Model file for the job. Use its own axes, mm. Face numbers are marked on the shaded views. A direction names the side the tool comes from. Round coordinates to 2 decimals unless told otherwise and drop trailing zeros. Loops run counter-clockwise (first coordinate to the right, second up) from the corner with the lowest first, then second, coordinate; pieces in that order, holes last. Notation, with made-up numbers: (60.25, -21) - (100.25, -21) arc R20 ccw to (100.25, 0) - close; hole circle Ø1 at (-16, 32.5). An arc over 180 degrees is marked (long way). Use one line per item in the form item = value.
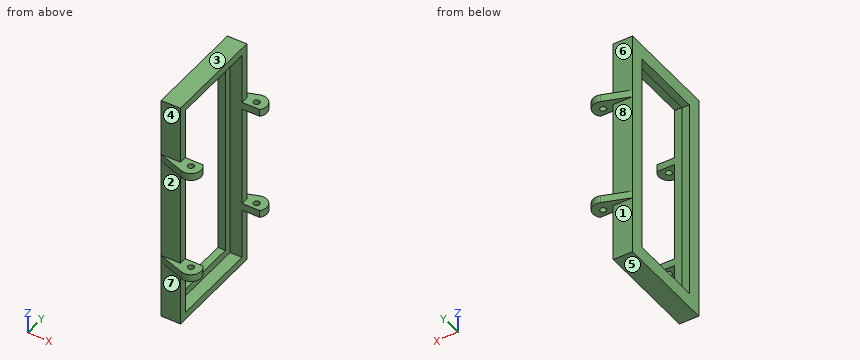
from build123d import *

# Parameters (mm, degrees)
SKETCH_1_W               = 114.4
SKETCH_1_H               = 50.4
SKETCH_1_W_2             = 107.2
SKETCH_1_H_2             = 43.2
SKETCH_1_W_3             = 100
SKETCH_1_H_3             = 36
EXTRUDE_1_DEPTH          = 3.6
SKETCH_1_3_W             = 114.4
SKETCH_1_3_H             = 50.4
SKETCH_1_3_W_2           = 107.2
SKETCH_1_3_H_2           = 43.2
EXTRUDE_2_DEPTH          = 9.5
EXTRUDE_START            = 25
SKETCH_2_R               = 1.5
EXTRUDE_3_DEPTH          = 3.6
MIRROR_START             = 25
MIRROR_2_COPY_1_SKETCH_R = 1.5
MIRROR_2_COPY_1_DEPTH    = 3.6


with BuildPart() as part:
    # Sketch 1 → Extrude 1 (new body)
    # profile 1 of 2: a face of its own
    with BuildSketch(Plane(origin=(0, 0, 0), x_dir=(0, 0, -1), z_dir=(1, 0, 0))):
        Rectangle(SKETCH_1_W, SKETCH_1_H)
        Rectangle(SKETCH_1_W_2, SKETCH_1_H_2, mode=Mode.SUBTRACT)
    # profile 2 of 2: a face of its own
    with BuildSketch(Plane(origin=(0, 0, 0), x_dir=(0, 0, -1), z_dir=(1, 0, 0))):
        Rectangle(SKETCH_1_W_2, SKETCH_1_H_2)
        Rectangle(SKETCH_1_W_3, SKETCH_1_H_3, mode=Mode.SUBTRACT)
    extrude(amount=EXTRUDE_1_DEPTH)

    # Sketch 1_3 → Extrude 2 (add)
    with BuildSketch(Plane(origin=(0, 0, 0), x_dir=(0, 0, -1), z_dir=(1, 0, 0))):
        Rectangle(SKETCH_1_3_W, SKETCH_1_3_H)
        Rectangle(SKETCH_1_3_W_2, SKETCH_1_3_H_2, mode=Mode.SUBTRACT)
    extrude(amount=EXTRUDE_2_DEPTH)

    # Sketch 2 → Extrude 3 (add)
    with BuildSketch(Plane.XY.offset(EXTRUDE_START)):
        with BuildLine():
            Line((12.840920286, 29.716720736), (0, 25.2))
            Line((0, 25.2), (0, 21.6))
            Line((0, 21.6), (9.5, 21.6))
            Line((9.5, 21.6), (18.166060556, 21.6))
            ThreePointArc((18.166060556, 21.6), (18.680583919, 27.74275739), (12.840920286, 29.716720736))
        make_face()
        with Locations((14.5, 25)):
            Circle(SKETCH_2_R, mode=Mode.SUBTRACT)
    extrude_3 = extrude(amount=EXTRUDE_3_DEPTH)

    # Mirror 1: Extrude 3 across plane
    add(extrude_3.mirror(Plane.XY))

    # Mirror 2: Extrude 3 across plane
    add(extrude_3.mirror(Plane.ZX))

    # Mirror 2 copy 1 sketch → Mirror 2 copy 1 (add)
    with BuildSketch(Plane(origin=(0, 0, 0), x_dir=(1, 0, 0), z_dir=(0, 0, -1)).offset(MIRROR_START)):
        with BuildLine():
            Line((12.840920286, 29.716720736), (0, 25.2))
            Line((0, 25.2), (0, 21.6))
            Line((0, 21.6), (9.5, 21.6))
            Line((9.5, 21.6), (18.166060556, 21.6))
            ThreePointArc((18.166060556, 21.6), (18.680583919, 27.74275739), (12.840920286, 29.716720736))
        make_face()
        with Locations((14.5, 25)):
            Circle(MIRROR_2_COPY_1_SKETCH_R, mode=Mode.SUBTRACT)
    extrude(amount=MIRROR_2_COPY_1_DEPTH)


solid = part.part
1. Cut at B-B, the plane x = 14.5. Give the number of separate pieces and of enclosed holes in the cut face, plus the area to 3 significant figures.
Geometry check:
separate_pieces = 8
enclosed_holes = 0
area = 77.8 mm^2
2. Pull direction Z, two halves, no side cores. Call the marked faces 1, 2 and 3: +Z half, -Z half, draft (parallel to the pull), parting line (faces both ways), or undercut.
Geometry check:
face_1 = draft
face_2 = undercut
face_3 = +Z half
3. Wall check: probe 1 along Y at (x, z) = (14.5, -25.95); probe 2 along Z at (x, y) = (1.25, 10); probe 3 along Y at (x, z) = (4, -13). Give the ranges that are in metal, low to high.
Geometry check:
probe_1 = -30 to -26.5, -23.5 to -21.6, 21.6 to 23.5, 26.5 to 30
probe_2 = -57.2 to -50, 50 to 57.2
probe_3 = -25.2 to -21.6, 21.6 to 25.2
4. Tool access for the marked faces 4, 5, 6, 7 and 8: list every direction of +Z, -Z, +X, -X, +Y, -Y with a clear straight run to the whole face (end or side of a thin tool).
Geometry check:
face_4 = +Z, +X, -X, -Y
face_5 = -Z, +X, -X, +Y, -Y
face_6 = +Z, +X, -X, +Y
face_7 = -Z, +X, -X, -Y
face_8 = +X, -X, +Y
5. Cut at A-A, the plane y = 6. Give the cut face in (x, z), plus the area to 3 significant figures.
Geometry check:
outline = (0, -57.2) - (9.5, -57.2) - (9.5, -53.6) - (3.6, -53.6) - (3.6, -50) - (0, -50) - close; (0, 50) - (3.6, 50) - (3.6, 53.6) - (9.5, 53.6) - (9.5, 57.2) - (0, 57.2) - close
area = 94.3 mm^2
6. Cut at C-C, the plane z = -48. Give the cut face in (x, y).
Geometry check:
outline = (0, -25.2) - (9.5, -25.2) - (9.5, -21.6) - (3.6, -21.6) - (3.6, -18) - (0, -18) - close; (0, 18) - (3.6, 18) - (3.6, 21.6) - (9.5, 21.6) - (9.5, 25.2) - (0, 25.2) - close
7. Flat gauge pins, fed straight in: pin 1 (10.5 mm diameter, centred on x = 6, z = -5.5, fed in from -Y); pin 2 (1.5 mm diameter, centred on y = 15.5, z = -30.5, fed in from +X) (3 decimals); pin 3 (23 mm diameter, centred on y = 9, z = 37, fed in from +X); pin 4 (1.1 mm diameter, centred on y = -24, z = -8.5, fed in from +X). Where does each tip first touch, or does it go through?
Geometry check:
pin_1 = -25.2
pin_2 = through
pin_3 = 3.6
pin_4 = 9.5
